Autodesk Inventor part; units mm, degrees
ref_plane "YZ Plane" through (0, 0, 0) normal (1, 0, 0) x (0, 1, 0)
ref_plane "XZ Plane" through (0, 0, 0) normal (0, 1, 0) x (-1, 0, 0)
ref_plane "XY Plane" through (0, 0, 0) normal (0, 0, 1) x (1, 0, 0)
sketch "Sketch1" plane through (0, 0, 0) normal (0, 1, 0) x (-1, 0, 0)
  line L0 (-5, 5) -> (5, 5) construction
  line L1 (5, 5) -> (5, -5) construction
  line L2 (5, -5) -> (-5, -5) construction
  line L3 (-5, -5) -> (-5, 5) construction
  line L4 (-5, 5) -> (5, -5) construction
  line L5 (5, 5) -> (-5, -5) construction
  line L6 (6.5, 22.5) -> (-6.5, 22.5)
  line L7 (-6.5, 22.5) -> (-6.5, -22.5)
  line L8 (-6.5, -22.5) -> (6.5, -22.5)
  line L9 (6.5, 22.5) -> (-6.5, -22.5) construction
  line L10 (-6.5, 22.5) -> (6.5, -22.5) construction
  arc A0 (6.5, -22.5) -> (6.5, 22.5) centre (-13.3431, 0) ccw
  point P0 (0, 0)
  dimension "d0" = 10
  dimension "d1" = 10
  dimension "d2" = 13
  dimension "d3" = 45
  dimension "d4" = 30
extrude "Extrusion1" add sketch "Sketch1" along normal blind 10
sketch "Sketch2" plane through (0, 0, 0) normal (0, -1, 0) x (1, 0, 0)
  line L0 (-5, 5) -> (5, 5)
  line L1 (5, 5) -> (5, -5)
  line L2 (5, -5) -> (-5, -5)
  line L3 (-5, -5) -> (-5, 5)
  line L4 (-5, 5) -> (5, -5) construction
  line L5 (5, 5) -> (-5, -5) construction
  point P0 (0, 0)
  dimension "d7" = 10
  dimension "d8" = 10
extrude "Extrusion2" add sketch "Sketch2" along normal blind 20
sketch "Sketch4" plane through (0, -20, 0) normal (0, -1, 0) x (1, 0, 0)
  line L0 (5, 5) -> (5, -5)
  line L1 (-5, 2.5) -> (5, 2.5)
  line L2 (5, 2.5) -> (5, -2.5)
  line L3 (5, -2.5) -> (-5, -2.5)
  line L4 (-5, -2.5) -> (-5, 2.5)
  line L5 (-5, 2.5) -> (5, -2.5) construction
  line L6 (5, 2.5) -> (-5, -2.5) construction
  line L7 (5, 5) -> (-5, 5)
  line L8 (-5, 5) -> (-5, -5)
  point P0 (0, 0)
  point P1 (5, 0)
  dimension "d11" = 5
  dimension "d14" = 10
extrude "Extrusion3" cut sketch "Sketch4" against normal blind 18 contours L0 L3 L4 L1
properties part number "holder_for_wire"
For this review, take the finished solid that the model builds, in its own axes (mm). A direction names the side the tool comes from. Coordinates: 2 decimals unless noted, no trailing zeros. Write each loop counter-clockwise with the first axis right and the second up, starting at its lowest first coordinate (ties: lowest second). Pieces come first, ordered by that corner, then holes.
(1) Add section A-A on y = -13.5. Give the boundary of the cut face in (x, z), then the cut area to 3 significant figures.
(2) Add section C-C on z = 0. Give the boundary of the cut face in (x, y), then the cut area to 3 significant figures.
(3) Tool access review of faces 1 (the face through (-5, -10, -3)), 2 (the face through (0, -11, 2.5)), 3 (the face through (0, -10, -5)), 4 (the face through (0, -10, 5)), 5 (the face through (5, -10, 3)): name each direction out of +Z, -Z, +X, -X, +Y, -Y from which nothing blocks a thin tool from reaching the whole face with its end or side.
(4) Add section D-D on y = 7.75. Give the boundary of the cut face in (x, z).
(5) Add section B-B on x = 1.5. Give the boundary of the cut face in (y, z), then the cut area to 3 significant figures.
(6) For pin 1 Ø5 at (x, y) = (1, -11) entering from -Z; pin 2 Ø4 at (x, z) = (-9, -5) entering from -Y; pin 3 Ø5 at (x, y) = (3, -13) entering from +Z, all flat-tipped, find the tip position at first contact; note any pin that passes through.
(7) The part is to be moulded in two halves that separate along Z. For faces 6 (the face through (0, -2, 0)), 7 (the face through (-16.655, 4.93, 0.356)), 8 (the face through (0, 5, -22.5)), 9 (the face through (0, -11, -2.5)), say which applies: +Z half, -Z half, draft (parallel to the pull), parting line (faces both ways), or undercut.
(8) Wall thickness on probe 1 along Z at (x, y) = (-2.75, -18.25); probe 2 along X at (y, z) = (-0.5, 4): over which ranges is each line inside the solid? List them lowest first.
Answer sheet:
1. outline: (-5, -5) - (5, -5) - (5, -2.5) - (-5, -2.5) - close; (-5, 2.5) - (5, 2.5) - (5, 5) - (-5, 5) - close
1. area: 50.0 mm2
2. outline: (-16.66, 0) - (-5, 0) - (-5, -2) - (5, -2) - (5, 0) - (6.5, 0) - (6.5, 10) - (-16.66, 10) - close
2. area: 252 mm2
3. face 1: +Z, -Z, -X, -Y
3. face 2: +X, -X, -Y
3. face 3: -Z, +X, -X, -Y
3. face 4: +Z, +X, -X, -Y
3. face 5: +Z, -Z, +X, -Y
4. outline: (-6.5, -22.5) - (6.5, -22.5) - (6.5, 22.5) - (-6.5, 22.5) arc R30 ccw to start
5. outline: (-20, -5) - (0, -5) - (0, -22.5) - (10, -22.5) - (10, 22.5) - (0, 22.5) - (0, 5) - (-20, 5) - (-20, 2.5) - (-2, 2.5) - (-2, -2.5) - (-20, -2.5) - close
5. area: 560 mm2
6. pin 1: stops at z = -5
6. pin 2: stops at y = 0
6. pin 3: stops at z = 5
7. face 6: undercut
7. face 7: parting line
7. face 8: -Z half
7. face 9: undercut
8. probe 1: z = -5 to -2.5, 2.5 to 5
8. probe 2: x = -5 to 5
